Verification items for the finished model (mm, model axes). Face numbers are marked on the shaded views. A direction names the side the tool comes from. Coordinates: 2 decimals unless noted, no trailing zeros. Write each loop counter-clockwise with the first axis right and the second up, starting at its lowest first coordinate (ties: lowest second). Pieces come first, ordered by that corner, then holes. Notation, with made-up numbers: (6, 74) -> (19, 74) arc R23 ccw to (19, 106) -> close; hole circle Ø2 at (-31, 14.25). An arc over 180 degrees is marked (long way). Answer in a Markdown table with one row per item.
```python
from build123d import *

# Parameters (mm, degrees)
BOSS_EXTRUDE1_DEPTH       = 48.26
SKETCH2_W                 = 3.175
SKETCH2_H                 = 25.298904356
BOSS_EXTRUDE2_DEPTH       = 19.05
TAP_DRILL_FOR_6_32_TAP1_D = 2.7051
TAP_DRILL_FOR_8_32_TAP1_D = 3.4544


with BuildPart() as part:
    # Sketch1 → Boss-Extrude1 (new body)
    with BuildSketch(Plane.XY):
        Polygon((15.875, 28.575), (-38.1, 28.575), (-38.1, 25.4), (0, 25.4), (0, 0), (3.175, 0), (3.175, 25.4), (15.875, 25.4), align=None)
    extrude(amount=BOSS_EXTRUDE1_DEPTH)

    # Sketch2 → Boss-Extrude2 (add)
    with BuildSketch(Plane(origin=(0, 28.575, 0), x_dir=(1, 0, 0), z_dir=(0, 1, 0))):
        with Locations((14.2875, -35.610547822)):
            Rectangle(SKETCH2_W, SKETCH2_H)
    extrude(amount=BOSS_EXTRUDE2_DEPTH)

    # Tap Drill for #6-32 Tap1 (through all)
    with Locations(Plane(origin=(15.875, 0, 0), x_dir=(0, 0, -1), z_dir=(1, 0, 0))):
        with Locations((-43.18, 38.735), (-30.48, 38.735)):
            Hole(TAP_DRILL_FOR_6_32_TAP1_D / 2)

    # Tap Drill for #8-32 Tap1 (through all)
    with Locations(Plane.ZY):
        with Locations((5.08, 12.7), (24.13, 12.7)):
            Hole(TAP_DRILL_FOR_8_32_TAP1_D / 2)


solid = part.part
```
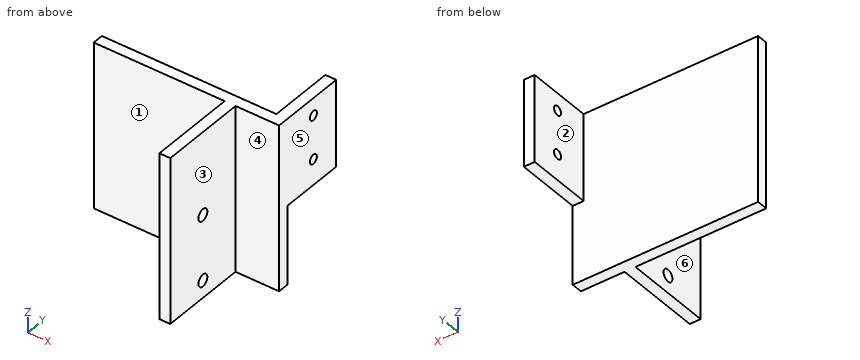
1. Sectioned sample at D-D, the plane z = 31. Record the cut outline in (x, y) (3 decimals), and give its area (3 significant figures).
Findings below:
| item | result |
|---|---|
| outline | (-38.1, 25.4) -> (0, 25.4) -> (0, 0) -> (3.175, 0) -> (3.175, 25.4) -> (15.875, 25.4) -> (15.875, 37.486) -> (12.7, 37.486) -> (12.7, 28.575) -> (-38.1, 28.575) -> close; (12.7, 39.984) -> (15.875, 39.984) -> (15.875, 47.625) -> (12.7, 47.625) -> close |
| area | 305 mm² |
2. Material ranges on probe 1 along Y at (x, z) = (14, 43) (3 decimals); probe 2 along Y at (x, z) = (-24.5, 4.5) (3 decimals); probe 3 along X at (y, z) = (7, 40) (3 decimals), recorded low to high. Write a range as from..to.
Findings below:
| item | result |
|---|---|
| probe 1 | y = 25.4..37.394, 40.076..47.625 |
| probe 2 | y = 25.4..28.575 |
| probe 3 | x = 0..3.175 |
3. Sectioned sample at B-B, the plane y = 12.7. Record the cut outline in (x, z) (3 decimals), and give its area (3 significant figures).
Findings below:
| item | result |
|---|---|
| outline | (0, 0) -> (3.175, 0) -> (3.175, 3.353) -> (0, 3.353) -> close; (0, 6.807) -> (3.175, 6.807) -> (3.175, 22.403) -> (0, 22.403) -> close; (0, 25.857) -> (3.175, 25.857) -> (3.175, 48.26) -> (0, 48.26) -> close |
| area | 131 mm² |
4. Sectioned sample at C-C, the plane z = 37.5. Record the cut outline in (x, y) (3 decimals).
Findings below:
| item | result |
|---|---|
| outline | (-38.1, 25.4) -> (0, 25.4) -> (0, 0) -> (3.175, 0) -> (3.175, 25.4) -> (15.875, 25.4) -> (15.875, 47.625) -> (12.7, 47.625) -> (12.7, 28.575) -> (-38.1, 28.575) -> close |
5. Access from +Z, -Z, +X, -X, +Y, -Y to the whole of each face (thin tool, end or side, straight path). Record for the marked faces 1, 2 and 3.
Findings below:
| item | result |
|---|---|
| face 1 | +Z, -Z, -X, -Y |
| face 2 | +Z, -Z, -X, +Y |
| face 3 | +Z, -Z, +X, -Y |
6. Release check for a two-part mould opening along X. For the marked faces 4, 5 and 6 record: released by +X, released by -X, zero draft, split by the parting line, or undercut.
Findings below:
| item | result |
|---|---|
| face 4 | zero draft |
| face 5 | released by +X |
| face 6 | released by -X |
7. Go/stop test with flat-tipped pins: pin 1 (2 mm diameter, centred on y = 12.7, z = 24.13, fed in from -X); pin 2 (2 mm diameter, centred on y = 5, z = 35, fed in from +X) (3 decimals); pin 3 (21 mm diameter, centred on y = 40, z = 31, fed in from -X); pin 4 (14.5 mm diameter, centred on x = -6.5, z = 34.5, fed in from +Y) (3 decimals). Record where each tip stops, or that it passes through.
Findings below:
| item | result |
|---|---|
| pin 1 | passes through |
| pin 2 | stops at x = 3.175 |
| pin 3 | stops at x = 12.7 |
| pin 4 | stops at y = 28.575 |
8. Sectioned sample at A-A, the plane z = 43.18. Record the cut outline in (x, y) (3 decimals), and give its area (3 significant figures).
Findings below:
| item | result |
|---|---|
| outline | (-38.1, 25.4) -> (0, 25.4) -> (0, 0) -> (3.175, 0) -> (3.175, 25.4) -> (15.875, 25.4) -> (15.875, 37.382) -> (12.7, 37.382) -> (12.7, 28.575) -> (-38.1, 28.575) -> close; (12.7, 40.088) -> (15.875, 40.088) -> (15.875, 47.625) -> (12.7, 47.625) -> close |
| area | 304 mm² |
